Autodesk Inventor part; units mm, degrees
ref_plane "YZ Plane" through (0, 0, 0) normal (1, 0, 0) x (0, 1, 0)
ref_plane "XZ Plane" through (0, 0, 0) normal (0, 1, 0) x (-1, 0, 0)
ref_plane "XY Plane" through (0, 0, 0) normal (0, 0, 1) x (1, 0, 0)
sketch "Sketch1" plane through (0, 0, 0) normal (0, 1, 0) x (-1, 0, 0)
  line L0 (0, 0) -> (0, -355.998) construction
  line L1 (5, 0) -> (5, -355.998)
  line L2 (-5, -355.998) -> (-5, 0)
  arc A0 (5, 0) -> (-5, 0) centre (0, 0) ccw
  arc A1 (-5, -355.998) -> (5, -355.998) centre (0, -355.998) ccw
  circle A2 centre (0, 0) radius 1.65
  circle A3 centre (0, -355.998) radius 1.65
  circle A4 centre (0, -57.376) radius 1.65
  point P0 (0, -177.999)
  dimension "d0" = 3.3
  dimension "d1" = 3.3
  dimension "d2" = 10
  dimension "d3" = 355.998
  dimension "d14" = 3.3
  dimension "d15" = 57.376
extrude "Extrusion1" add sketch "Sketch1" along normal blind 3
sketch "Sketch2" plane through (0, 3, 0) normal (0, 1, 0) x (1, 0, 0)
  line L0 (-26.2185, 378.6248) -> (37.2853, 378.6248)
  line L1 (37.2853, 378.6248) -> (37.2853, 176.2061)
  line L2 (37.2853, 176.2061) -> (-26.2185, 176.2061)
  line L3 (-26.2185, 176.2061) -> (-26.2185, 378.6248)
  line L4 (-95.1798, 405.4155) -> (74.9908, 405.4155)
  line L5 (74.9908, 405.4155) -> (74.9908, -44.073)
  line L6 (74.9908, -44.073) -> (-95.1798, -44.073)
  line L7 (-95.1798, -44.073) -> (-95.1798, 405.4155)
  point P0 (0, 0)
extrude "Extrusion2" cut sketch "Sketch2" against normal blind 10
properties part number "Part_10_p2"
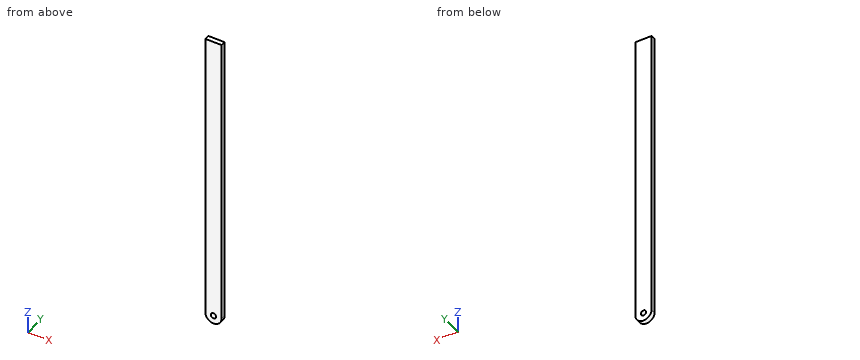
Design review of the part built by this model. Coordinates are the model's own, in mm. Round coordinates to 2 decimals unless told otherwise and drop trailing zeros. Write each loop counter-clockwise with the first axis right and the second up, starting at its lowest first coordinate (ties: lowest second). Pieces come first, ordered by that corner, then holes.
Item 1: For pin 1 Ø1 at (x, y) = (-3.5, 2) entering from -Z, flat-tipped, find the tip position at first contact; note if it passes through.
Item 2: Consider section A-A on x = 0. Give the boundary of the cut face in (y, z), and give its area (3 significant figures).
Item 3: Wall thickness on L1, parallel to Z at x = 0, y = 0.7; L2, parallel to Z at x = 1.5, y = 2.75; L3, parallel to Z at x = -2, y = 0.75: over which ranges is each line inside the solid? List them lowest first.
Check values:
1. pin 1: stops at z = -360
2. outline: (0, -361) - (3, -361) - (3, -357.65) - (0, -357.65) - close; (0, -354.35) - (3, -354.35) - (3, -176.21) - (0, -176.21) - close
2. area: 544 mm2
3. L1: z = -361 to -357.65, -354.35 to -176.21
3. L2: z = -360.77 to -356.69, -355.31 to -176.21
3. L3: z = -360.58 to -176.21
